Geometry check sheet. Reference: the model listing, model coordinates, mm. A direction names the side the tool comes from. Round coordinates to 2 decimals unless told otherwise and drop trailing zeros. One line per question, with ' | ' between items. Start each with the question number.
Q1. Gauge pin test, flat ends, axial feed: P1, Ø1.5, axis at x = 2, z = -52, coming from the +Y side; P2, Ø1, axis at x = 1.5, y = -4, coming from the -Z side; P3, Ø1.5, axis at x = 1, y = 96, coming from the -Z side. Record the tip position at first contact, or that the pin passes through.
Q2. Sectioned sample at A-A, the plane x = 0.75. Give the number of separate pieces and of enclosed holes in the cut face, then the cut area to 3 significant figures.
Q3. Material ranges on line 1 along Y through (x, z) = (2.95, -41.87); line 2 along Y through (x, z) = (2.3, -211.5); line 3 along Y through (x, z) = (3.75, -40), recorded low to high.
Q4. Mould release check, pull along Z, two halves, no side actions. Record for faces 1 (the face through (2.46, 70.54, -114.24)), 2 (the face through (2.465, 90.667, 1.269)), 3 (the face through (2.465, -10.879, 126.155)): +Z half, -Z half, draft (parallel to the pull), parting line (faces both ways), or undercut.
Q5. Tool access check on faces 4 (the face through (5, 25, -50)), 5 (the face through (2.46, 56.74, -128.42)). Record the directions out of +Z, -Z, +X, -X, +Y, -Y that give a thin tool (end or side, any length) a straight path to the whole face; none if there is none.
```python
from build123d import *

# Parameters (mm, degrees)
SCHIZZO3_R                   = 1.5
ESTRUSIONE_ESTRUSIONE1_DEPTH = 5
SCHIZZO2_R                   = 2
SCHIZZO2_R_2                 = 9.75
TAGLIO_ESTRUSIONE1_DEPTH     = 6
TAGLIO_ESTRUSIONE2_DEPTH     = 6
SCHIZZO6_R                   = 1.5
SCHIZZO6_R_2                 = 4
SCHIZZO6_W                   = 5
SCHIZZO6_H                   = 15
SCHIZZO6_H_2                 = 12.5
TAGLIO_ESTRUSIONE3_DEPTH     = 6
SCHIZZO7_R                   = 1.5
TAGLIO_ESTRUSIONE4_DEPTH     = 6


with BuildPart() as part:
    # Schizzo3 → Estrusione-Estrusione1 (new body)
    with BuildSketch(Plane(origin=(0, 0, 0), x_dir=(0, 0, -1), z_dir=(1, 0, 0))):
        with BuildLine():
            Line((-95, -33), (201, -33))
            ThreePointArc((201, -33), (233.396512744, -6.282194046), (213.334616938, 30.608123513))
            Line((213.334616938, 30.608123513), (12.334616938, 111.608123513))
            ThreePointArc((12.334616938, 111.608123513), (-5.305430843, 113.570729245), (-21.410737295, 106.111358555))
            Line((-21.410737295, 106.111358555), (-116.410737295, 25.111358555))
            ThreePointArc((-116.410737295, 25.111358555), (-125.96509997, -11.408881796), (-95, -33))
        make_face()
        with Locations((-65.666686189, 61.806607259)):
            Circle(SCHIZZO3_R, mode=Mode.SUBTRACT)
        with Locations((110.965735584, 66.470529041)):
            Circle(SCHIZZO3_R, mode=Mode.SUBTRACT)
        with Locations((73.86497981, 81.421579875)):
            Circle(SCHIZZO3_R, mode=Mode.SUBTRACT)
        with Locations((148.066491357, 51.519478207)):
            Circle(SCHIZZO3_R, mode=Mode.SUBTRACT)
    extrude(amount=ESTRUSIONE_ESTRUSIONE1_DEPTH)

    # Schizzo2 → Taglio-Estrusione1 (cut, through all)
    with BuildSketch(Plane(origin=(0, 0, 0), x_dir=(0, 0, -1), z_dir=(1, 0, 0))):
        with Locations((-95, 0)):
            Circle(SCHIZZO2_R)
        with Locations((201, 0)):
            Circle(SCHIZZO2_R)
        with Locations((12.990381057, 73.5)):
            Circle(SCHIZZO2_R)
        with Locations((-12.990381057, 73.5)):
            Circle(SCHIZZO2_R)
        with Locations((0, 96)):
            Circle(SCHIZZO2_R)
        with Locations((0, 81)):
            Circle(SCHIZZO2_R_2)
    extrude(amount=TAGLIO_ESTRUSIONE1_DEPTH, mode=Mode.SUBTRACT)

    # Schizzo4 → Taglio-Estrusione2 (cut, through all)
    with BuildSketch(Plane(origin=(0, 0, 0), x_dir=(0, 0, -1), z_dir=(1, 0, 0))):
        Polygon((104.943784553, 71.592648309), (103.074903199, 66.955053837), (79.886930841, 76.299460608), (81.755812195, 80.93705508), align=None)
        Polygon((118.856567968, 65.986004246), (116.987686614, 61.348409774), (140.175658973, 52.004003003), (142.044540327, 56.641597475), align=None)
        Polygon((-82.507716927, 50.732778486), (-72.995838686, 58.842906249), (-69.751787581, 55.038154953), (-79.263665822, 46.92802719), align=None)
        Polygon((-61.581584798, 68.575059565), (-58.337533692, 64.770308269), (-48.825655452, 72.880436032), (-52.069706557, 76.685187328), align=None)
    extrude(amount=TAGLIO_ESTRUSIONE2_DEPTH, mode=Mode.SUBTRACT)

    # Schizzo6 → Taglio-Estrusione3 (cut, through all)
    with BuildSketch(Plane(origin=(5, 0, 0), x_dir=(0, 0, -1), z_dir=(1, 0, 0))):
        with Locations((41.87, 15.17)):
            Circle(SCHIZZO6_R)
        with Locations((-58.13, 15.17)):
            Circle(SCHIZZO6_R)
        with Locations((141.87, 15.17)):
            Circle(SCHIZZO6_R)
        with Locations((53, -15)):
            Circle(SCHIZZO6_R_2)
        with Locations((53, 20.84)):
            Circle(SCHIZZO6_R)
        with Locations((41.87, -3)):
            Rectangle(SCHIZZO6_W, SCHIZZO6_H)
        with Locations((41.87, 33.34)):
            Rectangle(SCHIZZO6_W, SCHIZZO6_H)
        with Locations((141.87, 33.34)):
            Rectangle(SCHIZZO6_W, SCHIZZO6_H)
        with Locations((141.87, -3)):
            Rectangle(SCHIZZO6_W, SCHIZZO6_H)
        with Locations((-58.13, -3)):
            Rectangle(SCHIZZO6_W, SCHIZZO6_H)
        with Locations((-58.13, 33.34)):
            Rectangle(SCHIZZO6_W, SCHIZZO6_H)
        with Locations((53, 34.59)):
            Rectangle(SCHIZZO6_W, SCHIZZO6_H_2)
        with Locations((53, 7.09)):
            Rectangle(SCHIZZO6_W, SCHIZZO6_H_2)
    extrude(amount=-TAGLIO_ESTRUSIONE3_DEPTH, mode=Mode.SUBTRACT)

    # Schizzo7 → Taglio-Estrusione4 (cut, through all)
    with BuildSketch(Plane(origin=(0, 0, 0), x_dir=(0, 0, -1), z_dir=(1, 0, 0))):
        with Locations((-95, 7)):
            Circle(SCHIZZO7_R)
        with Locations((-90, 7)):
            Circle(SCHIZZO7_R)
        with Locations((-85, 7)):
            Circle(SCHIZZO7_R)
        with Locations((-80, 7)):
            Circle(SCHIZZO7_R)
        with Locations((-100, 7)):
            Circle(SCHIZZO7_R)
        with Locations((-105, 7)):
            Circle(SCHIZZO7_R)
        with Locations((-110, 7)):
            Circle(SCHIZZO7_R)
        with Locations((-80, -7)):
            Circle(SCHIZZO7_R)
        with Locations((-85, -7)):
            Circle(SCHIZZO7_R)
        with Locations((-90, -7)):
            Circle(SCHIZZO7_R)
        with Locations((-95, -7)):
            Circle(SCHIZZO7_R)
        with Locations((-100, -7)):
            Circle(SCHIZZO7_R)
        with Locations((-105, -7)):
            Circle(SCHIZZO7_R)
        with Locations((-110, -7)):
            Circle(SCHIZZO7_R)
        with Locations((216, -7)):
            Circle(SCHIZZO7_R)
        with Locations((211, -7)):
            Circle(SCHIZZO7_R)
        with Locations((206, -7)):
            Circle(SCHIZZO7_R)
        with Locations((201, -7)):
            Circle(SCHIZZO7_R)
        with Locations((196, -7)):
            Circle(SCHIZZO7_R)
        with Locations((191, -7)):
            Circle(SCHIZZO7_R)
        with Locations((186, -7)):
            Circle(SCHIZZO7_R)
        with Locations((186, 7)):
            Circle(SCHIZZO7_R)
        with Locations((191, 7)):
            Circle(SCHIZZO7_R)
        with Locations((196, 7)):
            Circle(SCHIZZO7_R)
        with Locations((201, 7)):
            Circle(SCHIZZO7_R)
        with Locations((206, 7)):
            Circle(SCHIZZO7_R)
        with Locations((211, 7)):
            Circle(SCHIZZO7_R)
        with Locations((216, 7)):
            Circle(SCHIZZO7_R)
        with BuildLine():
            Line((-105, 2), (-85, 2))
            ThreePointArc((-85, 2), (-83, 0), (-85, -2))
            Line((-85, -2), (-105, -2))
            ThreePointArc((-105, -2), (-107, 0), (-105, 2))
        make_face()
        with BuildLine():
            Line((191, 2), (211, 2))
            ThreePointArc((211, 2), (213, 0), (211, -2))
            Line((211, -2), (191, -2))
            ThreePointArc((191, -2), (189, 0), (191, 2))
        make_face()
    extrude(amount=TAGLIO_ESTRUSIONE4_DEPTH, mode=Mode.SUBTRACT)


solid = part.part
```
Determined:
1) P1: stops at y = 95.93 | P2: stops at z = -233.81 | P3: stops at z = -52.93
2) separate pieces: 1 | enclosed holes: 55 | area: 34,700 mm2
3) line 1: y = -33 to -10.5, 4.5 to 13.67, 16.67 to 25.84, 40.84 to 99.71 | line 2: y = -31.28 to -8.41, -5.59 to -1.94, 1.94 to 5.59, 8.41 to 31.35 | line 3: y = -33 to -10.5, 4.5 to 25.84, 40.84 to 100.46
4) face 1: -Z half | face 2: undercut | face 3: +Z half
5) face 4: +Z, -Z, +X, +Y, -Y | face 5: +X, -X
